The model under review builds one solid part; all positions refer to its coordinate system, in mm. A direction names the side the tool comes from. Give positions to 0.01 mm unless a question says otherwise; leave off trailing zeros. Loops run counter-clockwise (first coordinate to the right, second up) from the corner with the lowest first, then second, coordinate; pieces in that order, holes last. Notation, with made-up numbers: M 37,83.25 L 92,83.25 A15 cw 92,92.25 Z; hole C -16.5,16.25 d8. An arc over 180 degrees is marked long. Return JSON: item names as keys, results as strings. Group by question number.
```python
from build123d import *

# Parameters (mm, degrees)
CROQUIS1_R              = 3.5
SALIENTE_EXTRUIR1_DEPTH = 16
CROQUIS2_W              = 18.232700604
CROQUIS2_H              = 9.1
CORTAR_EXTRUIR1_DEPTH   = 22
CROQUIS3_R              = 3.5
CROQUIS3_R_2            = 2.65
SALIENTE_EXTRUIR2_DEPTH = 1.5
SALIENTE_EXTRUIR3_START = -1.5
CROQUIS4_R              = 3.5
CROQUIS4_R_2            = 2.65
SALIENTE_EXTRUIR3_DEPTH = 1.5
CROQUIS5_R              = 4.5
SALIENTE_EXTRUIR4_DEPTH = 2.5


with BuildPart() as part:
    # Croquis1 → Saliente-Extruir1 (new body)
    with BuildSketch(Plane.XY):
        with BuildLine():
            Line((-19.490709772, 9.428309156), (-7.90572953, 9.428309156))
            ThreePointArc((-7.90572953, 9.428309156), (-3.938516352, 6.040037718), (1.230212675, 5.330528037))
            Line((1.230212675, 5.330528037), (1.314384466, 5.340636055))
            ThreePointArc((1.314384466, 5.340636055), (5.463239212, -0.634836445), (0.054718216, -5.499727804))
            ThreePointArc((0.054718216, -5.499727804), (-12.283781153, -1.395117758), (-19.490709772, 9.428309156))
        make_face()
        Circle(CROQUIS1_R, mode=Mode.SUBTRACT)
    extrude(amount=SALIENTE_EXTRUIR1_DEPTH)

    # Croquis2 → Cortar-Extruir1 (cut)
    with BuildSketch(Plane(origin=(0, 9.428309156, 0), x_dir=(1, 0, 0), z_dir=(0, 1, 0))):
        with Locations((1.210620772, -8)):
            Rectangle(CROQUIS2_W, CROQUIS2_H)
    extrude(amount=-CORTAR_EXTRUIR1_DEPTH, mode=Mode.SUBTRACT)

    # Croquis3 → Saliente-Extruir2 (add)
    with BuildSketch(Plane(origin=(0, 0, 12.55), x_dir=(-1, 0, 0), z_dir=(0, 0, -1))):
        Circle(CROQUIS3_R)
        Circle(CROQUIS3_R_2, mode=Mode.SUBTRACT)
    extrude(amount=-SALIENTE_EXTRUIR2_DEPTH)

    # Croquis4 → Saliente-Extruir3 (add)
    with BuildSketch(Plane.XY.offset(3.45).offset(SALIENTE_EXTRUIR3_START)):
        Circle(CROQUIS4_R)
        with Locations(Location((0, 0, 0), (0, 0, 180))):
            Circle(CROQUIS4_R_2, mode=Mode.SUBTRACT)
    extrude(amount=SALIENTE_EXTRUIR3_DEPTH)

    # Croquis5 → Saliente-Extruir4 (add)
    with BuildSketch(Plane(origin=(0, 9.428309156, 0), x_dir=(1, 0, 0), z_dir=(0, 1, 0))):
        with Locations(Location((-13.698219651, -8, 0), (0, 0, 270))):
            Circle(CROQUIS5_R)
    extrude(amount=SALIENTE_EXTRUIR4_DEPTH)


solid = part.part
```
(1) Add section D-D (z = 7). Write out the cut boundary in (x, y), and give its area (3 significant figures).
(2) For faces 4 (the cylindrical face through (3.233, -1.341, 0.961)), 5 (the cylindrical face through (-12.347, 10.661, 12.292)), 6 (the flat face through (-3, 0, 3.45)), 7 (the flat face through (-7, 2, 0)), 8 (the flat face through (1, 3, 14.05)), list the 3-axis set-ups (+Z, -Z, +X, -X, +Y, -Y) from which the entire face can be reached by the end or side of a thin tool; tool diameter is ignored.
(3) For probe 1 along Z at (x, y) = (-2, -2); probe 2 along Y at (x, z) = (0, 15.6); probe 3 along Y at (x, z) = (0, 13), list the stretches that pass through material, from the lowest coordinate up.
(4) Add section C-C (x = -4.75). Write out the cut boundary in (y, z).
(5) Add section B-B (z = 15). Write out the cut boundary in (x, y), and give its area (3 significant figures).
(6) For pin 1 (2.5 mm diameter, centred on y = 6, z = 8.5, fed in from +X); pin 2 (3 mm diameter, centred on y = 4.5, z = 14, fed in from -X); pin 3 (1 mm diameter, centred on y = 7.5, z = 4, fed in from -X), all flat-tipped, find the tip position at first contact; note any pin that passes through.
(7) Mouldability with a two-part tool opening along Y and no side actions: class faces 1 (the flat face through (-7.906, 3, 8)), 2 (the cylindrical face through (3.233, -1.341, 15.011)), 3 (the cylindrical face through (5.475, -0.524, 14.251)) as released by +Y, released by -Y, zero draft, split by the parting line, or undercut.
(8) Add section A-A (y = -2.25). Write out the cut boundary in (x, z), and give its area (3 significant figures).
Verdict:
{
 "1": {"outline": "M -19.49,9.43 A20 ccw -7.91,-3.93 L -7.91,9.43 L -9.31,9.43 L -9.31,11.93 L -18.09,11.93 L -18.09,9.43 Z", "area": "124 mm²"},
 "2": {"face 4": "-Z", "face 5": "+Y", "face 6": "+X, +Y, -Y", "face 7": "-Z, +X, -X, +Y, -Y", "face 8": "+Z"},
 "3": {"probe 1": "z = 1.95 to 3.45, 12.55 to 14.05", "probe 2": "y = -5.5 to -3.5, 3.5 to 5.23", "probe 3": "y = -5.5 to -2.65, 2.65 to 5.23"},
 "4": {"outline": "M -4.96,0 L 6.45,0 L 6.45,3.45 L -4.96,3.45 Z; M -4.96,12.55 L 6.45,12.55 L 6.45,16 L -4.96,16 Z"},
 "5": {"outline": "M -19.49,9.43 A20 ccw 0.05,-5.5 A5.5 ccw 1.31,5.34 L 1.23,5.33 A9.27 cw -7.91,9.43 Z; hole C 0,0 d7", "area": "201 mm²"},
 "6": {"pin 1": "stops at x = -7.91", "pin 2": "stops at x = -18.25", "pin 3": "stops at x = -19.06"},
 "7": {"face 1": "zero draft", "face 2": "undercut", "face 3": "split by the parting line"},
 "8": {"outline": "M -11.07,0 L -2.68,0 L -2.68,1.95 L -1.4,1.95 L -1.4,3.45 L -7.91,3.45 L -7.91,12.55 L -1.4,12.55 L -1.4,14.05 L -2.68,14.05 L -2.68,16 L -11.07,16 Z; M 1.4,1.95 L 2.68,1.95 L 2.68,0 L 5.02,0 L 5.02,3.45 L 1.4,3.45 Z; M 1.4,12.55 L 5.02,12.55 L 5.02,16 L 2.68,16 L 2.68,14.05 L 1.4,14.05 Z", "area": "111 mm²"}
}
